Study the drawing (mm; zero at the part's minimum x, y, z) and answer. A direction names the side the tool comes from. Coordinates: 2 decimals unless noted, no trailing zeros. Loops run counter-clockwise (first coordinate to the right, second up) from the corner with the lowest first, then second, coordinate; pieces in that order, holes last.
Q1. The mould has two halves that part along Z. Classify the marked faces 4, 5, 6 and 7: pulls with the +Z half, pulls with the -Z half, needs draft (parallel to the pull), parting line crosses it, or undercut.
Q2. Straight lines are drawn through the part: line 1 (Z direction, x = 38.1, y = 2.75); line 2 (X direction, y = 8.5, z = 6.5) (1 decimal); line 3 (X direction, y = 10, z = 25) (1 decimal). For each, find the intervals that lie inside material, in ascending order.
Q3. Flat-ended cylindrical pins translate along their axes: P1, Ø5, axis at x = 12, z = 24, coming from the -Y side; P2, Ø9, axis at x = 38.1, z = 9.525, coming from the +Y side; P3, Ø4, axis at x = 18.5, y = 9, coming from the +Z side; P4, Ø1, axis at y = 10.5, z = 34.5, coming from the -X side. Find the tip coordinate at first contact, or state that the pin passes through.
Q4. Section A-A (y = 10.5) is taken. Count the separate pieces of the cut face and the enclosed holes in it, then the cut area to 3 significant figures.
Q5. Section B-B (x = 38.1) is taken. Give the vertices of the cut face in (y, z), then the cut area to 3 significant figures.
Q6. Which of the six approach directions +Z, -Z, +X, -X, +Y, -Y give full straight-line access (tool end or side, diameter ignored) to the marked faces 1, 2 and 3?
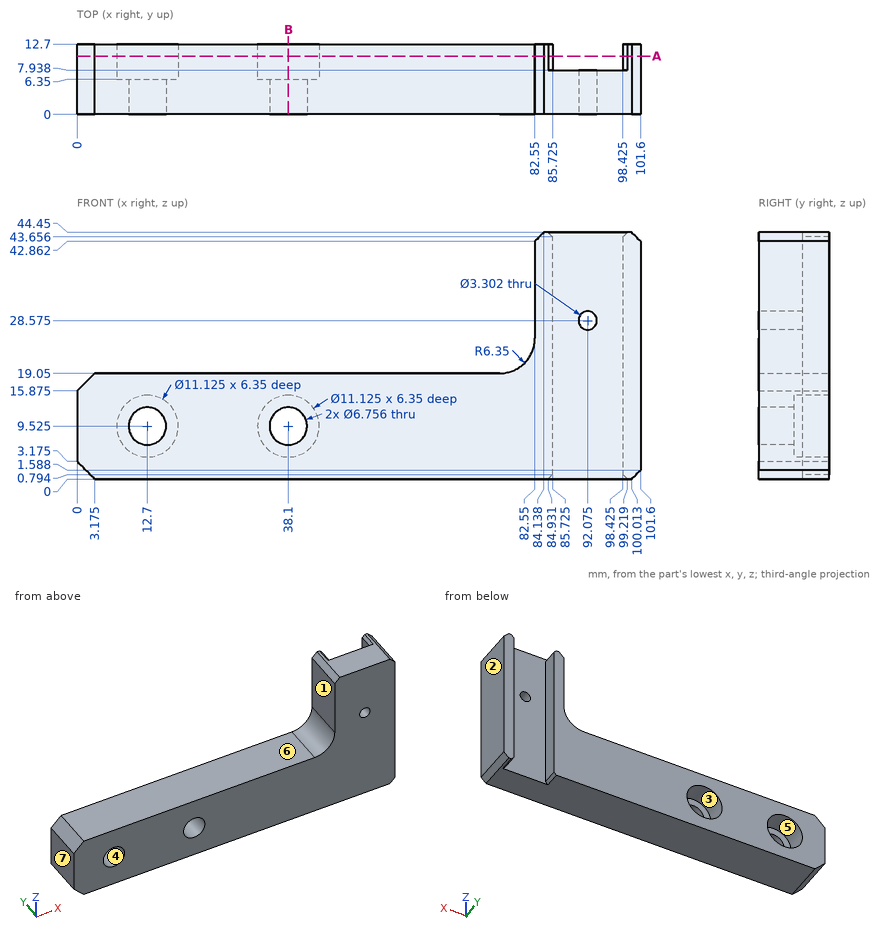
Numbers:
1. face 4: undercut
1. face 5: undercut
1. face 6: pulls with the +Z half
1. face 7: needs draft
2. line 1: z = 0 to 6.15, 12.9 to 19.05
2. line 2: x = 0 to 8, 17.4 to 33.4, 42.8 to 85.7, 98.4 to 101.6
2. line 3: x = 82.5 to 85.7, 98.4 to 101.6
3. P1: passes through
3. P2: stops at y = 6.35
3. P3: stops at z = 19.05
3. P4: stops at x = 82.55
4. separate pieces: 2
4. enclosed holes: 2
4. area: 1,650 mm2
5. outline: (0, 0) - (12.7, 0) - (12.7, 3.96) - (6.35, 3.96) - (6.35, 6.15) - (0, 6.15) - close; (0, 12.9) - (6.35, 12.9) - (6.35, 15.09) - (12.7, 15.09) - (12.7, 19.05) - (0, 19.05) - close
5. area: 128 mm2
6. face 1: +Z, -X, +Y, -Y
6. face 2: +Z, -Z, +X, +Y, -Y
6. face 3: +Y
